For this review, take the finished solid that the model builds, in its own axes (mm). A direction names the side the tool comes from. Give positions to 0.01 mm unless a question says otherwise; leave off trailing zeros. Loops run counter-clockwise (first coordinate to the right, second up) from the corner with the lowest first, then second, coordinate; pieces in that order, holes last. Notation, with made-up numbers: (38.5, -11) - (52.5, -11) arc R25 cw to (52.5, 8) - close; hole circle Ø5 at (-21.5, 12). An arc over 180 degrees is marked (long way). Put each result on its own line as item: value.
Autodesk Inventor part; units mm, degrees
ref_plane "YZ Plane" through (0, 0, 0) normal (1, 0, 0) x (0, 1, 0)
ref_plane "XZ Plane" through (0, 0, 0) normal (0, 1, 0) x (-1, 0, 0)
ref_plane "XY Plane" through (0, 0, 0) normal (0, 0, 1) x (1, 0, 0)
sketch "Sketch1" plane through (0, 0, 0) normal (0, 0, 1) x (1, 0, 0)
  line L0 (0, 0) -> (60, 0)
  line L1 (60, 0) -> (60, 100)
  line L2 (60, 100) -> (0, 100)
  line L3 (0, 100) -> (0, 0)
  line L4 (-5, 0) -> (65, 0)
  line L5 (65, 0) -> (65, 105)
  line L6 (65, 105) -> (-5, 105)
  line L7 (-5, 105) -> (-5, 0)
  dimension "d0" = 60
  dimension "d1" = 100
  dimension "d2" = 5
  dimension "d3" = 5
  dimension "d4" = 5
extrude "Extrusion1" add sketch "Sketch1" along normal blind 14
sketch "Sketch2" plane through (-5, 0, 0) normal (0, -1, 0) x (1, 0, 0)
  line L0 (5, 2) -> (65, 2)
  line L1 (65, 2) -> (65, 12)
  line L2 (65, 12) -> (5, 12)
  line L3 (5, 12) -> (5, 2)
  line L4 (0, 14) -> (70, 14)
  line L5 (0, 0) -> (70, 0)
  line L6 (70, 0) -> (70, 14)
  line L7 (0, 0) -> (0, 14)
  point P0 (5, 0)
  dimension "d7" = 2
  dimension "d8" = 2
  dimension "d9" = 5
  dimension "d10" = 5
extrude "Extrusion2" cut sketch "Sketch2" against normal blind 103 contours L3 L2 L1 L0
sketch "Sketch3" plane through (0, 0, 14) normal (0, 0, 1) x (1, 0, 0)
  line L0 (37.75, 103) -> (22.25, 103)
  line L1 (22.25, 103) -> (22.25, 82)
  line L2 (22.25, 82) -> (37.75, 82)
  line L3 (37.75, 82) -> (37.75, 103)
  line L4 (65, 105) -> (-5, 105)
  line L5 (0, 0) -> (0, 103)
  line L6 (0, 103) -> (60, 103)
  line L7 (0, 103) -> (60, 103)
  line L8 (60, 0) -> (60, 103)
  line L9 (22.25, 103) -> (22.25, 105)
  line L10 (65, 105) -> (-5, 105)
  line L11 (37.75, 103) -> (37.75, 105)
  line L12 (22.25, 105) -> (37.75, 105)
  dimension "d13" = 2
  dimension "d14" = 22.25
  dimension "d15" = 15.5
  dimension "d16" = 21
  dimension "d17" = 60
  dimension "d18" = 22.25
extrude "Extrusion3" cut sketch "Sketch3" against normal up to surface (14 mm away)
sketch "Sketch4" plane through (65, 0, 0) normal (1, 0, 0) x (0, 0, -1)
  circle A0 centre (-7, 78) radius 2
  circle A1 centre (-7, 35) radius 2
  line L0 (-12, 103) -> (-2, 103)
  line L1 (-12, 0) -> (-12, 103)
  line L2 (0, 0) -> (-14, 0)
  dimension "d21" = 4
  dimension "d22" = 4
  dimension "d23" = 25
  dimension "d24" = 5
  dimension "d25" = 35
  dimension "d26" = 5
extrude "Extrusion4" cut sketch "Sketch4" against normal up to surface (42.75 mm away)
properties part number "Heatsink Jig"
1) Insertion check: pin 1 Ø2 at (x, z) = (28.5, 0.5) entering from +Y; pin 2 Ø3 at (x, z) = (45, 8) entering from -Y. Each pin has a flat end and moves straight along its axis. Give the tip position at first contact, or say it passes through.
Geometry check:
pin 1: stops at y = 82
pin 2: stops at y = 103
2) Take a section at A-A on z = 7. State the section outline as (x, y) points.
Geometry check:
outline: (-5, 0) - (0, 0) - (0, 103) - (22.25, 103) - (22.25, 105) - (-5, 105) - close; (37.75, 103) - (60, 103) - (60, 80) - (65, 80) - (65, 105) - (37.75, 105) - close; (60, 0) - (65, 0) - (65, 33) - (60, 33) - close; (60, 37) - (65, 37) - (65, 76) - (60, 76) - close
3) Draft analysis for pull direction X (two halves, no side actions). For faces 4 (the face through (63, 80, 7)), 5 (the face through (22.25, 95.3, 12.2)), 6 (the face through (-5, 53, 7)), state which applies: pulls with the +X half, pulls with the -X half, needs draft (parallel to the pull), parting line crosses it, or undercut.
Geometry check:
face 4: needs draft
face 5: undercut
face 6: pulls with the -X half
4) Take a section at B-B on x = 30. State the section outline as (y, z) points, and give its area (3 significant figures).
Geometry check:
outline: (0, 0) - (82, 0) - (82, 2) - (0, 2) - close; (0, 12) - (82, 12) - (82, 14) - (0, 14) - close
area: 328 mm²
5) For faces 1 (the face through (49, 103, 7)), 2 (the face through (63, 33, 7)), 3 (the face through (30, 82, 1)), list the 3-axis set-ups (+Z, -Z, +X, -X, +Y, -Y) from which the entire face can be reached by the end or side of a thin tool; tool diameter is ignored.
Geometry check:
face 1: -Y
face 2: +X
face 3: +Z, -Z, +Y
6) Take a section at C-C on y = 35. State the section outline as (x, z) points.
Geometry check:
outline: (-5, 0) - (65, 0) - (65, 5) - (60, 5) - (60, 2) - (0, 2) - (0, 12) - (60, 12) - (60, 9) - (65, 9) - (65, 14) - (-5, 14) - close
7) Wall thickness on line 1 (Y direction, x = 62.5, z = 7); line 2 (X direction, y = 91.5, z = 9.5); line 3 (Z direction, x = 19.5, y = 50.5): over which ranges is each line inside the solid? List them lowest first.
Geometry check:
line 1: y = 0 to 33, 37 to 76, 80 to 105
line 2: x = -5 to 0, 60 to 65
line 3: z = 0 to 2, 12 to 14
8) Take a section at D-D on x = 20. State the section outline as (y, z) points, and give its area (3 significant figures).
Geometry check:
outline: (0, 0) - (105, 0) - (105, 14) - (0, 14) - (0, 12) - (103, 12) - (103, 2) - (0, 2) - close
area: 440 mm²
